```python
from build123d import *

# Parameters (mm, degrees)
F1_DEPTH = 63.5
F2_DEPTH = 25.4


# Not quite as in the source:
# - a feature of the source that left no trace in its solid (it failed there, or was rolled back) is left out


with BuildPart() as f1:
    # F0 (on Front) → F1 (new body, symmetric)
    with BuildSketch(Plane.XZ):
        Polygon((22.225, 12.7436925435), (-41.275, 12.7436925435), (-41.275, -6.3063074565), (41.275, -6.3063074565), (41.275, 12.7436925435), align=None)
    extrude(amount=F1_DEPTH, both=True)

    # F0 (on Front) → F2 (join, symmetric)
    with BuildSketch(Plane.XZ):
        with BuildLine():
            Line((22.225, 30.2188925435), (22.225, 12.7436925435))
            Line((22.225, 12.7436925435), (41.275, 12.7436925435))
            Line((41.275, 12.7436925435), (41.275, 30.2188925435))
            ThreePointArc((41.275, 30.2188925435), (45.9246798487, 41.4442126948), (57.15, 46.0938925435))
            Line((57.15, 46.0938925435), (60.325, 46.0938925435))
            Line((60.325, 46.0938925435), (60.325, 65.1438925435))
            Line((60.325, 65.1438925435), (57.15, 65.1438925435))
            add(Edge.make_bspline(
                [(57.15, 65.1438925435), (56.7668826582, 65.1373961276), (56.3837003417, 65.1310994591), (56.0004776373, 65.1249697126)],
                knots=[0, 0, 0, 0, 0.9177220122, 0.9177220122, 0.9177220122, 0.9177220122], degree=3))
            ThreePointArc((56.0004776373, 65.1249697126), (32.0511684185, 54.5047789437), (22.225, 30.2188925435))
        make_face()
    extrude(amount=F2_DEPTH, both=True)


solid = f1.part
```
Input: part model. Units: mm. Frame: model coordinates. A direction names the side the tool comes from. Give positions to 0.01 mm unless a question says otherwise; leave off trailing zeros. Loops run counter-clockwise (first coordinate to the right, second up) from the corner with the lowest first, then second, coordinate; pieces in that order, holes last.
1) Reachability of faces 1 (the flat face through (22.225, 0, 22)), 2 (the flat face through (37, 25.4, 39)), 3 (the flat face through (59, 0, 46.094)), 4 (the flat face through (37, -25.4, 39)) from +Z, -Z, +X, -X, +Y, -Y: full face, straight path, thin tool, end or side. Return the list, or none.
A:
face 1: +Z, -X, +Y, -Y
face 2: +Z, +X, -X, +Y
face 3: -Z, +X, +Y, -Y
face 4: +Z, +X, -X, -Y
2) Section query A-A on z = 21. Return the cut outline in (x, y) (3 decimals), and give its area (3 significant figures).
A:
outline: (22.225, -25.4) - (41.275, -25.4) - (41.275, 25.4) - (22.225, 25.4) - close
area: 968 mm2
3) Section query B-B on x = -22. Return the cut outline in (y, z), and give its area (3 significant figures).
A:
outline: (-63.5, -6.31) - (63.5, -6.31) - (63.5, 12.74) - (-63.5, 12.74) - close
area: 2,420 mm2
4) Line query: L1, parallel to Z at x = -25.5, y = 38; L2, parallel to X at y = 49, z = 12.5 (3 decimals); L3, parallel to X at y = -24.5, z = 30 (3 decimals). Output: solid intervals per line, ascending.
A:
L1: z = -6.31 to 12.74
L2: x = -41.275 to 41.275
L3: x = 22.225 to 41.275
5) Contact query for flat-ended pins moving along their axis: pin 1 (18.5 mm diameter, centred on y = 7, z = 9, fed in from +X) (3 decimals); pin 2 (4 mm diameter, centred on y = 26.5, z = 51.5, fed in from -X); pin 3 (19 mm diameter, centred on x = 38.5, z = 47, fed in from -Y); pin 4 (5 mm diameter, centred on y = -38.5, z = 16, fed in from +X). Output: stop coordinate, or through.
A:
pin 1: stops at x = 41.275
pin 2: stops at x = 28.25
pin 3: stops at y = -25.4
pin 4: passes through
